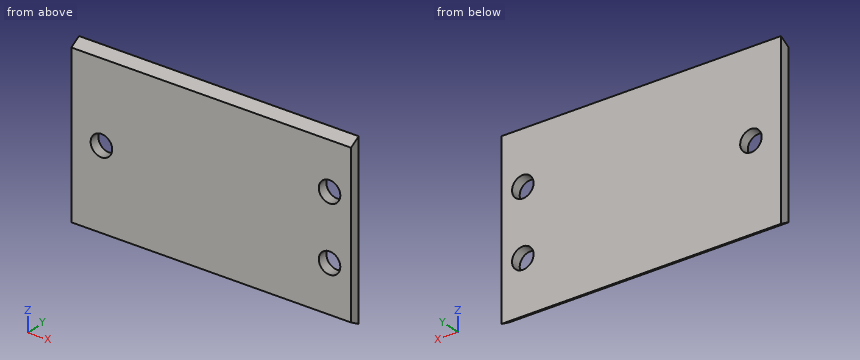
```python
from build123d import *

# Parameters (mm, degrees)
SKETCH1_W           = 32.5
SKETCH1_H           = 20
SKETCH1_R           = 1.25
BOSS_EXTRUDE1_DEPTH = 1.2
CHAMFER1_SIZE       = 1.2
CHAMFER1_SIZE_2     = 0.692820323
CHAMFER2_SIZE       = 1.2
CHAMFER2_SIZE_2     = 0.692820323


with BuildPart() as part:
    # Sketch1 → Boss-Extrude1 (new body)
    with BuildSketch(Plane(origin=(0, 0, 0), x_dir=(1, 0, 0), z_dir=(0, 1, 0))):
        with Locations((16.25, 10)):
            Rectangle(SKETCH1_W, SKETCH1_H)
        with Locations(Location((30, 6.2, 0), (0, 0, 270))):
            Circle(SKETCH1_R, mode=Mode.SUBTRACT)
        with Locations(Location((30, 13.8, 0), (0, 0, 270))):
            Circle(SKETCH1_R, mode=Mode.SUBTRACT)
        with Locations(Location((3.5, 10, 0), (0, 0, 270))):
            Circle(SKETCH1_R, mode=Mode.SUBTRACT)
    extrude(amount=-BOSS_EXTRUDE1_DEPTH)

    # Chamfer1
    # the kernel refuses this chamfer: 1.2, 0.692820323 mm, written as the material it takes off along each edge
    with BuildSketch(Plane(origin=(35.604502906, -1.2, -20), x_dir=(0, 0.9998132206222078, -0.019326765612701437), z_dir=(-1, 0, 0))) as chamfer1_piece_1:
        Polygon((CHAMFER1_SIZE * 0.999813220622, -CHAMFER1_SIZE * 0.0193267656127), (-CHAMFER1_SIZE_2 * 0.0193267656135, -CHAMFER1_SIZE_2 * 0.999813220662), (0, 0), align=None)
    extrude(amount=38.709005811, mode=Mode.SUBTRACT)

    # Chamfer2
    # the kernel refuses this chamfer: 1.2, 0.692820323 mm, written as the material it takes off along each edge
    with BuildSketch(Plane(origin=(-3.104502906, -1.2, 0), x_dir=(0, 0.999813220622208, 0.01932676561270074), z_dir=(1, 0, 0))) as chamfer2_piece_1:
        Polygon((CHAMFER2_SIZE * 0.999813220622, -CHAMFER2_SIZE * 0.0193267656127), (-CHAMFER2_SIZE_2 * 0.0193267656135, -CHAMFER2_SIZE_2 * 0.999813220662), (0, 0), align=None)
    extrude(amount=38.709005811, mode=Mode.SUBTRACT)


solid = part.part
```
The model under review builds one solid part; all positions refer to its coordinate system, in mm. Give positions to 0.01 mm unless a question says otherwise; leave off trailing zeros. Loops run counter-clockwise (first coordinate to the right, second up) from the corner with the lowest first, then second, coordinate; pieces in that order, holes last. Notation, with made-up numbers: (-33, 63.25) - (-21, 63.25) arc R28 ccw to (-21, 84.25) - close; hole circle Ø10 at (50, 33.5). An arc over 180 degrees is marked (long way). Answer as a JSON object with one key per item and string values.
Q1. Add section D-D on x = 24. State the section outline as (y, z) points.
Worked out:
{"outline": "(-1.2, -19.31) - (0, -20) - (0, 0) - (-1.2, -0.69) - close"}
Q2. Add section B-B on x = 3.5. State the section outline as (y, z) points.
Worked out:
{"outline": "(-1.2, -19.31) - (0, -20) - (0, -11.25) - (-1.2, -11.25) - close; (-1.2, -8.75) - (0, -8.75) - (0, 0) - (-1.2, -0.69) - close"}
Q3. Add section C-C on y = -0.3. State the section outline as (x, z) points.
Worked out:
{"outline": "(0, -19.83) - (32.5, -19.83) - (32.5, -0.17) - (0, -0.17) - close; hole circle Ø2.5 at (3.5, -10); hole circle Ø2.5 at (30, -13.8); hole circle Ø2.5 at (30, -6.2)"}
Q4. Add section A-A on z = -13.8. State the section outline as (x, y) points, plus the area to 3 significant figures.
Worked out:
{"outline": "(0, -1.2) - (28.75, -1.2) - (28.75, 0) - (0, 0) - close; (31.25, -1.2) - (32.5, -1.2) - (32.5, 0) - (31.25, 0) - close", "area": "36.0 mm^2"}
Q5. Insertion check: pin 1 (2 mm diameter, centred on x = 30, z = -13.8, fed in from +Y). The pin has a flat end and moves straight along its axis. Give the tip position at first contact, or say it passes through.
Worked out:
{"pin 1": "passes through"}
Q6. To check wall thickness, follow line 1 along X through (y, z) = (-0.7, -6.2); line 2 along X through (y, z) = (-0.3, -10); line 3 along Z through (x, y) = (31, -0.25). State the ranges of each line that lie inside material, in increasing order.
Worked out:
{"line 1": "x = 0 to 28.75, 31.25 to 32.5", "line 2": "x = 0 to 2.25, 4.75 to 32.5", "line 3": "z = -19.86 to -14.55, -13.05 to -6.95, -5.45 to -0.14"}
